```python
from build123d import *

# Parameters (mm, degrees)
SKETCH1_W           = 9.398
SKETCH1_H           = 9.398
BOSS_EXTRUDE1_DEPTH = 23.876
SKETCH2_W           = 14.478
SKETCH2_H           = 4.826
CUT_EXTRUDE1_DEPTH  = 10.398
SKETCH3_R           = 2.413
CUT_EXTRUDE2_DEPTH  = 10.398
SKETCH4_R           = 2.413
BOSS_EXTRUDE2_DEPTH = 101.6


with BuildPart() as part:
    # Sketch1 → Boss-Extrude1 (new body)
    with BuildSketch(Plane.XY):
        Rectangle(SKETCH1_W, SKETCH1_H)
    extrude(amount=BOSS_EXTRUDE1_DEPTH)

    # Sketch2 → Cut-Extrude1 (cut, through all)
    with BuildSketch(Plane(origin=(4.699, 0, 0), x_dir=(0, 0, -1), z_dir=(1, 0, 0))):
        with Locations((-16.637, 0)):
            Rectangle(SKETCH2_W, SKETCH2_H)
    extrude(amount=-CUT_EXTRUDE1_DEPTH, mode=Mode.SUBTRACT)

    # Sketch3 → Cut-Extrude2 (cut, through all)
    with BuildSketch(Plane(origin=(0, 4.699, 0), x_dir=(1, 0, 0), z_dir=(0, 1, 0))):
        with Locations((0, -19.177)):
            Circle(SKETCH3_R)
    extrude(amount=-CUT_EXTRUDE2_DEPTH, mode=Mode.SUBTRACT)

    # Sketch4 → Boss-Extrude2 (add)
    with BuildSketch(Plane(origin=(0, 0, 0), x_dir=(-1, 0, 0), z_dir=(0, 0, -1))):
        Circle(SKETCH4_R)
    extrude(amount=BOSS_EXTRUDE2_DEPTH)


solid = part.part
```
For this review, take the finished solid that the model builds, in its own axes (mm). A direction names the side the tool comes from. Round coordinates to 2 decimals unless told otherwise and drop trailing zeros. Loops run counter-clockwise (first coordinate to the right, second up) from the corner with the lowest first, then second, coordinate; pieces in that order, holes last.
(1) Mouldability with a two-part tool opening along X and no side actions: class faces 4 (the cylindrical face through (1.915, -1.468, -50.089)), 5 (the cylindrical face through (1.297, -3.54, 17.142)), 6 (the flat face through (1.1, 2.413, 16.7)) as released by +X, released by -X, zero draft, split by the parting line, or undercut.
Returned:
face 4: split by the parting line
face 5: undercut
face 6: zero draft
(2) We need section A-A (x = 0). Give the boundary of the cut face in (y, z), plus the area to 3 significant figures.
Returned:
outline: (-4.7, 0) - (-2.41, 0) - (-2.41, -101.6) - (2.41, -101.6) - (2.41, 0) - (4.7, 0) - (4.7, 16.76) - (2.41, 16.76) - (2.41, 9.4) - (-2.41, 9.4) - (-2.41, 16.76) - (-4.7, 16.76) - close; (-4.7, 21.59) - (-2.41, 21.59) - (-2.41, 23.88) - (-4.7, 23.88) - close; (2.41, 21.59) - (4.7, 21.59) - (4.7, 23.88) - (2.41, 23.88) - close
area: 623 mm2
(3) We need section B-B (y = 0). Give the boundary of the cut face in (x, z), plus the area to 3 significant figures.
Returned:
outline: (-4.7, 0) - (-2.41, 0) - (-2.41, -101.6) - (2.41, -101.6) - (2.41, 0) - (4.7, 0) - (4.7, 9.4) - (-4.7, 9.4) - close
area: 579 mm2
(4) Wall thickness on line 1 along Z through (x, y) = (0, 3.2); line 2 along Z through (x, y) = (-2.5, -3.5); line 3 along Z through (x, y) = (0.75, 1.5): over which ranges is each line inside the solid? List them lowest first.
Returned:
line 1: z = 0 to 16.76, 21.59 to 23.88
line 2: z = 0 to 23.88
line 3: z = -101.6 to 9.4
(5) Clearance check with flat-ended pins moving along their axes: P1, Ø1.5, axis at x = -2, y = 2, coming from the +Z side; P2, Ø1, axis at x = -1.5, z = -37, coming from the -Y side; P3, Ø1, axis at y = -1.5, z = -50.5, coming from the +X side; P4, Ø1.5, axis at x = 3.5, y = -2, coming from the -Z side. State where each tip first meets the part, or that it passes through.
Returned:
P1: stops at z = 23.88
P2: stops at y = -2.2
P3: stops at x = 2.2
P4: stops at z = 0
(6) We need section C-C (z = -26.5). Give the boundary of the cut face in (x, y), plus the area to 3 significant figures.
Returned:
outline: circle Ø4.83 at (0, 0)
area: 18.3 mm2
(7) Tool access review of faces 1 (the flat face through (-2, 2, 0)), 2 (the flat face through (0, 4, 23.876)), 3 (the flat face through (0, 0, 9.398)): name each direction out of +Z, -Z, +X, -X, +Y, -Y from which nothing blocks a thin tool from reaching the whole face with its end or side.
Returned:
face 1: -Z
face 2: +Z, +X, -X, +Y, -Y
face 3: +Z, +X, -X
